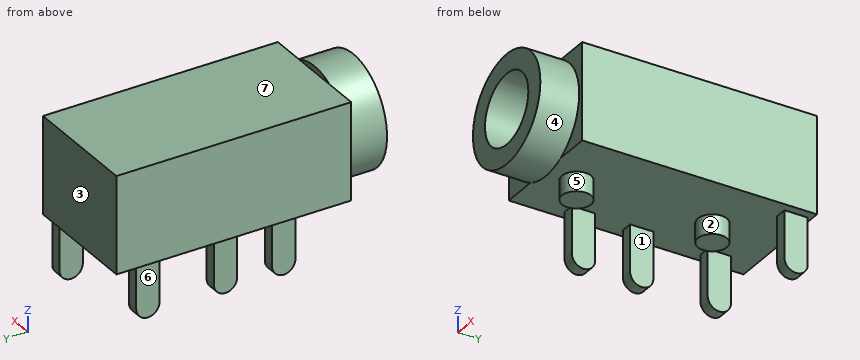
from build123d import *

# Parameters (mm, degrees)
SKETCH1_W           = 6.1
SKETCH1_H           = 12.1
BOSS_EXTRUDE1_DEPTH = 5
SKETCH2_R           = 2.8
SKETCH2_R_2         = 1.8
BOSS_EXTRUDE2_DEPTH = 2
SKETCH3_R           = 0.75
BOSS_EXTRUDE3_DEPTH = 1
SKETCH4_W           = 0.6
SKETCH4_H           = 1.2
BOSS_EXTRUDE4_DEPTH = 3
FILLET1_R           = 0.6


with BuildPart() as part:
    # Sketch1 → Boss-Extrude1 (new body)
    with BuildSketch(Plane.XY):
        Rectangle(SKETCH1_W, SKETCH1_H)
    extrude(amount=BOSS_EXTRUDE1_DEPTH)

    # Sketch2 → Boss-Extrude2 (add)
    with BuildSketch(Plane.XZ.offset(6.05)):
        with Locations(Location((0, 2.5, 0), (0, 0, 63.234499423))):
            Circle(SKETCH2_R)
        with Locations(Location((0, 2.5, 0), (0, 0, 270))):
            Circle(SKETCH2_R_2, mode=Mode.SUBTRACT)
    extrude(amount=BOSS_EXTRUDE2_DEPTH)

    # Sketch3 → Boss-Extrude3 (add)
    with BuildSketch(Plane(origin=(0, 0, 0), x_dir=(-1, 0, 0), z_dir=(0, 0, -1))):
        with Locations(Location((0, -4.45, 0), (0, 0, 180))):
            Circle(SKETCH3_R)
        with Locations(Location((0, 2.55, 0), (0, 0, 180))):
            Circle(SKETCH3_R)
    extrude(amount=BOSS_EXTRUDE3_DEPTH)

    # Sketch4 → Boss-Extrude4 (add)
    with BuildSketch(Plane(origin=(0, 0, 0), x_dir=(-1, 0, 0), z_dir=(0, 0, -1))):
        with Locations((2.3, -2.85)):
            Rectangle(SKETCH4_W, SKETCH4_H)
        with Locations((2.3, 0.15)):
            Rectangle(SKETCH4_W, SKETCH4_H)
        with Locations((2.3, 4.15)):
            Rectangle(SKETCH4_W, SKETCH4_H)
        with Locations((-2.3, 5.25)):
            Rectangle(SKETCH4_W, SKETCH4_H)
    extrude(amount=BOSS_EXTRUDE4_DEPTH)

    # Fillet1
    fillet1_edges = [part.edges().sort_by_distance(p)[0] for p in [
        (-2.3, 4.75, -3),
        (2.3, 5.85, -3),
        (2.3, 4.65, -3),
        (-2.3, 3.55, -3),
        (-2.3, 0.75, -3),
        (-2.3, -0.45, -3),
        (-2.3, -2.25, -3),
        (-2.3, -3.45, -3),
    ]]
    fillet(fillet1_edges, radius=FILLET1_R - 0.0001)  # a hair under: the kernel refuses the full size


solid = part.part
Build history of the part. All positions in model axes, mm. Face numbers are marked on the shaded views. A direction names the side the tool comes from. Give positions to 0.01 mm unless a question says otherwise; leave off trailing zeros. Order: outer loops, then holes, each group sorted by start corner. A loop starts at its lowest first (then second) coordinate and runs counter-clockwise, first axis right, second up. Notation, with made-up numbers: M 15.25,-39 L 27.25,-39 A22 ccw 27.25,-9 Z; hole C -5,-26 d7. An arc over 180 degrees is marked long. Use one line per item in the form item = value.
Q1. Pin check, flat tips, straight feed: P1, Ø0.5, axis at x = -2.5, z = -0.5, coming from the -Y side; P2, Ø2, axis at x = -1.5, z = 2, coming from the -Y side; P3, Ø0.6, axis at y = -3, z = -1.5, coming from the +X side; P4, Ø3, axis at y = -1, z = -2, coming from the -X side. Stop position of each tip, or through.
Conclusion:
P1 = -3.45
P2 = -8.05
P3 = -2
P4 = -2.6
Q2. Slice it at A-A, the plane z = -1.25. Write the cut outline in (x, y).
Conclusion:
outline = M -2.6,-3.45 L -2,-3.45 L -2,-2.25 L -2.6,-2.25 Z; M -2.6,-0.45 L -2,-0.45 L -2,0.75 L -2.6,0.75 Z; M -2.6,3.55 L -2,3.55 L -2,4.75 L -2.6,4.75 Z; M 2,4.65 L 2.6,4.65 L 2.6,5.85 L 2,5.85 Z
Q3. Slice it at C-C, the plane x = 0. Write the cut outline in (y, z).
Conclusion:
outline = M -8.05,-0.3 L -6.05,-0.3 L -6.05,0 L -5.2,0 L -5.2,-1 L -3.7,-1 L -3.7,0 L 1.8,0 L 1.8,-1 L 3.3,-1 L 3.3,0 L 6.05,0 L 6.05,5 L -6.05,5 L -6.05,5.3 L -8.05,5.3 L -8.05,4.3 L -6.05,4.3 L -6.05,0.7 L -8.05,0.7 Z
Q4. Pull direction Y, two halves, no side cores. Call the marked faces 1, 2 and 3: released by +Y, released by -Y, zero draft, split by the parting line, or undercut.
Conclusion:
face_1 = zero draft
face_2 = undercut
face_3 = released by +Y
Q5. Which spindle directions (+Z, -Z, +X, -X, +Y, -Y) get a long thin tool onto all of the face, cutting with end or side? Do the marked faces 4, 5, 6 and 7. Say none if no direction does.
Conclusion:
face_4 = -Y
face_5 = -Z
face_6 = -Z, -X, +Y, -Y
face_7 = +Z, +X, -X, +Y
Q6. Slice it at D-D, the plane z = 2.5. Write the cut outline in (x, y), and give its area (3 significant figures).
Conclusion:
outline = M -3.05,-6.05 L -2.8,-6.05 L -2.8,-8.05 L -1.8,-8.05 L -1.8,-6.05 L 1.8,-6.05 L 1.8,-8.05 L 2.8,-8.05 L 2.8,-6.05 L 3.05,-6.05 L 3.05,6.05 L -3.05,6.05 Z
area = 77.8 mm2
Q7. Slice it at B-B, the plane y = 2.55. Write the cut outline in (x, z), and give its area (3 significant figures).
Conclusion:
outline = M -3.05,0 L -0.75,0 L -0.75,-1 L 0.75,-1 L 0.75,0 L 3.05,0 L 3.05,5 L -3.05,5 Z
area = 32.0 mm2
Q8. Wall check: probe 1 along Y at (x, z) = (-2.5, -1); probe 2 along X at (y, z) = (-6.65, 2.5); probe 3 along Y at (x, z) = (3, 4.25). Give the ranges that are in metal, low to high.
Conclusion:
probe_1 = -3.45 to -2.25, -0.45 to 0.75, 3.55 to 4.75
probe_2 = -2.8 to -1.8, 1.8 to 2.8
probe_3 = -6.05 to 6.05
